Geometry check sheet. Reference: the model listing, model coordinates, mm. A direction names the side the tool comes from. Round coordinates to 2 decimals unless told otherwise and drop trailing zeros. Write each loop counter-clockwise with the first axis right and the second up, starting at its lowest first coordinate (ties: lowest second). Pieces come first, ordered by that corner, then holes. Notation, with made-up numbers: (78, 34.25) -> (109, 34.25) arc R5 cw to (109, 43.25) -> close; hole circle Ø7 at (65.25, -13.75). An arc over 180 degrees is marked (long way). Use a Markdown table: item, result.
```python
from build123d import *

# Parameters (mm, degrees)
PAD_DEPTH       = 25
SKETCH001_R     = 13
POCKET_DEPTH    = 61.214203
SKETCH002_R     = 0.8
POCKET001_DEPTH = 6


with BuildPart() as part:
    # Sketch → Pad (new body)
    with BuildSketch(Plane.XY):
        Polygon((0, 21.213203), (-21.213203, 21.213203), (0, 0), (0, -5), (4, -5), (4, -15), (0, -15), (0, -20), (20, -20), (20, 41.213203), (0, 41.213203), (0, 36.213203), (4, 36.213203), (4, 26.213203), (0, 26.213203), align=None)
    extrude(amount=PAD_DEPTH)

    # Sketch001 (on Face1 of Pad) → Pocket (cut, through all)
    with BuildSketch(Plane(origin=(0, 41.213203, 0), x_dir=(-1, 0, 0), z_dir=(0, 1, 0))):
        with Locations((-18, 12.5)):
            Circle(SKETCH001_R)
    extrude(amount=-POCKET_DEPTH, mode=Mode.SUBTRACT)

    # Sketch002 (on Face13 of Pocket) → Pocket001 (cut)
    with BuildSketch(Plane(origin=(0, 0, 0), x_dir=(0.707107, -0.707107, 0), z_dir=(-0.707107, -0.707107, 0))):
        with Locations((-25, 23)):
            Circle(SKETCH002_R)
        with Locations((-25, 2)):
            Circle(SKETCH002_R)
        with Locations((-12.5, 23)):
            Circle(SKETCH002_R)
        with Locations((-12.5, 2)):
            Circle(SKETCH002_R)
    extrude(amount=-POCKET001_DEPTH, mode=Mode.SUBTRACT)


solid = part.part
```
(1) Section check D-D on z = 4.25. Record the cut outline in (x, y), plus the area to 3 significant figures.
A:
| item | result |
|---|---|
| outline | (-21.21, 21.21) -> (0, 0) -> (0, -5) -> (4, -5) -> (4, -15) -> (0, -15) -> (0, -20) -> (7.95, -20) -> (7.95, 41.21) -> (0, 41.21) -> (0, 36.21) -> (4, 36.21) -> (4, 26.21) -> (0, 26.21) -> (0, 21.21) -> close |
| area | 632 mm2 |
(2) Section check B-B on y = -10. Record the cut outline in (x, z), plus the area to 3 significant figures.
A:
| item | result |
|---|---|
| outline | (4, 0) -> (14.43, 0) arc R13 cw to (14.43, 25) -> (4, 25) -> close |
| area | 86.9 mm2 |
(3) Release check for a two-part mould opening along Y. For faces 1 (the face through (4, 41.213, 12)), 2 (the face through (2, 36.213, 12)), 3 (the face through (4, 11, 0)), 4 (the face through (-11, 11, 12)) record: +Y half, -Y half, draft (parallel to the pull), parting line (faces both ways), or undercut.
A:
| item | result |
|---|---|
| face 1 | +Y half |
| face 2 | undercut |
| face 3 | draft |
| face 4 | -Y half |
(4) Access from +Z, -Z, +X, -X, +Y, -Y to the whole of each face (thin tool, end or side, straight path). Record for faces 5 (the face through (0, -17, 12)), 6 (the face through (4, -10, 12)), 7 (the face through (-4.604, 13.089, 2.011)).
A:
| item | result |
|---|---|
| face 5 | +Z, -Z, -X, -Y |
| face 6 | +Z, -Z, -X |
| face 7 | none |
(5) Section check A-A on z = 8. Record the cut outline in (x, y).
A:
| item | result |
|---|---|
| outline | (-21.21, 21.21) -> (0, 0) -> (0, -5) -> (4, -5) -> (4, -15) -> (0, -15) -> (0, -20) -> (5.8, -20) -> (5.8, 41.21) -> (0, 41.21) -> (0, 36.21) -> (4, 36.21) -> (4, 26.21) -> (0, 26.21) -> (0, 21.21) -> close |
(6) Section check C-C on x = -11. Record the cut outline in (y, z), plus the area to 3 significant figures.
A:
| item | result |
|---|---|
| outline | (11, 0) -> (21.21, 0) -> (21.21, 25) -> (11, 25) -> close |
| area | 255 mm2 |
(7) Thickness scan on line 1 (Y direction, x = 3, z = 13); line 2 (Z direction, x = 10, y = 4); line 3 (Y direction, x = -4.5, z = 23). Record the ranges inside material, lowest first.
A:
| item | result |
|---|---|
| line 1 | y = -20 to -15, -5 to 26.21, 36.21 to 41.21 |
| line 2 | z = 0 to 2.25, 22.75 to 25 |
| line 3 | y = 4.5 to 12.05, 12.99 to 21.21 |
(8) Gauge pin test, flat ends, axial feed: pin 1 Ø1.5 at (y, z) = (38.5, 10.5) entering from -X; pin 2 Ø1 at (x, y) = (-10, 8.5) entering from -Z; pin 3 Ø3 at (y, z) = (33, 14.5) entering from -X; pin 4 Ø10.5 at (x, z) = (-5.5, 7) entering from +Y. Record the tip position at first contact, or that the pin passes through.
A:
| item | result |
|---|---|
| pin 1 | stops at x = 0 |
| pin 2 | passes through |
| pin 3 | stops at x = 4 |
| pin 4 | stops at y = 21.21 |
